For this review, take the finished solid that the model builds, in its own axes (mm). Face numbers are marked on the shaded views. A direction names the side the tool comes from. Give positions to 0.01 mm unless a question says otherwise; leave off trailing zeros. Write each loop counter-clockwise with the first axis right and the second up, starting at its lowest first coordinate (ties: lowest second). Pieces come first, ordered by that corner, then holes.
1) For P1, Ø1.1, axis at x = -0.5, y = 10.5, coming from the -Z side; P2, Ø1, axis at x = -8, y = 10.5, coming from the -Z side; P3, Ø5, axis at y = 7.5, z = 1, coming from the +X side, all flat-tipped, find the tip position at first contact; note any pin that passes through.
2) Machinability: for the marked faces 1, 2 and 3, which of the approach directions +Z, -Z, +X, -X, +Y, -Y give a long, thin tool a straight path to every point of the face, cutting with its end or side? Answer none if there is none.
3) Wall thickness on line 1 along Y through (x, z) = (0, 1.2); line 2 along Z through (x, y) = (-3.25, 2); line 3 along Y through (x, z) = (-12, 11): over which ranges is each line inside the solid? List them lowest first.
4) Draft analysis for pull direction X (two halves, no side actions). For the marked faces 4, 5, 6 and 7, state which applies: pulls with the +X half, pulls with the -X half, needs draft (parallel to the pull), parting line crosses it, or undercut.
5) We need section A-A on z = 20.5. Give the boundary of the cut face in (x, y), and give its area (3 significant figures).
from build123d import *

# Parameters (mm, degrees)
F0_R     = 13.97
F1_DEPTH = 16.51
F2_R     = 7.62
F3_R     = 1.27
F4_DEPTH = 2.54
F5_R     = 1.905
F6_DEPTH = 2.54
F7_R     = 2.5019
F8_DEPTH = 12.7
F9_R     = 0.508


with BuildPart() as f1:
    # F0 (on Top) → F1 (new body)
    with BuildSketch(Plane.XY):
        Circle(F0_R)
    extrude(amount=F1_DEPTH)

    # F2
    f2_edges = [f1.edges().sort_by_distance(p)[0] for p in [
        (-13.97, 0, 16.51),
    ]]
    fillet(f2_edges, radius=F2_R)

    # F3 (on face) → F4 (join)
    with BuildSketch(Plane(origin=(0, 0, 0), x_dir=(1, 0, 0), z_dir=(0, 0, -1))):
        Circle(F3_R)
    extrude(amount=F4_DEPTH)

    # F5 (on face) → F6 (cut)
    with BuildSketch(Plane(origin=(0, 0, 0), x_dir=(1, 0, 0), z_dir=(0, 0, -1))):
        with Locations((-9.5885, 0)):
            Circle(F5_R)
        with Locations((0, -9.5885)):
            Circle(F5_R)
        with Locations((9.5885, 0)):
            Circle(F5_R)
        with Locations((0, 9.5885)):
            Circle(F5_R)
    extrude(amount=-F6_DEPTH, mode=Mode.SUBTRACT)

    # F7 (on face) → F8 (join)
    with BuildSketch(Plane.XY.offset(16.51)):
        Circle(F7_R)
    extrude(amount=F8_DEPTH)

    # F9
    f9_edges = [f1.edges().sort_by_distance(p)[0] for p in [
        (-2.5019, 0, 29.21),
    ]]
    fillet(f9_edges, radius=F9_R)


solid = f1.part
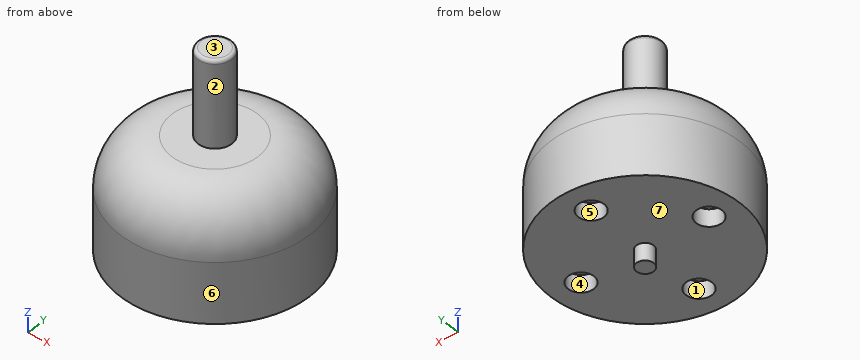
Results list:
1. P1: stops at z = 2.54
1. P2: stops at z = 0
1. P3: stops at x = 13.04
2. face 1: -Z
2. face 2: +Z
2. face 3: +Z, +X, -X, +Y, -Y
3. line 1: y = -13.97 to -11.49, -7.68 to 7.68, 11.49 to 13.97
3. line 2: z = 0 to 16.51
3. line 3: y = -6.55 to 6.55
4. face 4: undercut
4. face 5: undercut
4. face 6: parting line crosses it
4. face 7: needs draft
5. outline: circle Ø5 at (0, 0)
5. area: 19.7 mm2
